Part model, mm, in its own coordinate system. A direction names the side the tool comes from. Give positions to 0.01 mm unless a question says otherwise; leave off trailing zeros. Order: outer loops, then holes, each group sorted by start corner. A loop starts at its lowest first (then second) coordinate and runs counter-clockwise, first axis right, second up. Notation, with made-up numbers: (77.25, -10) -> (135.25, -10) arc R26 cw to (135.25, 25) -> close; hole circle Ø10 at (4, 54.25). An arc over 180 degrees is marked (long way). Write item = value, one per line. Start each with the question number.
Item 1: Band-saw the part on C-C on z = 0. Write the cut outline in (x, y).
Item 2: Band-saw the part on A-A on y = 0. Write the cut outline in (x, z), plus the area to 3 significant figures.
Item 3: Pull direction Z, two halves, no side cores. Call faces 1 (the face through (29, 0, 0)), 2 (the face through (14, -5, 0)), 3 (the face through (14.703, 3.797, 15.859)): +Z half, -Z half, draft (parallel to the pull), parting line (faces both ways), or undercut.
Item 4: Band-saw the part on D-D on z = 8.5. Write the cut outline in (x, y).
Item 5: Tool access for faces 4 (the face through (31.96, -1.15, 5.73)), 5 (the face through (-1.5, -0.1, 2.5)), 6 (the face through (14.703, 3.797, -15.859)): list every direction of +Z, -Z, +X, -X, +Y, -Y with a clear straight run to the whole face (end or side of a thin tool).
Item 6: Flat gauge pins, fed straight in: P1, Ø1, axis at y = 1, z = -5, coming from the -X side; P2, Ø3, axis at x = 15, y = 3.5, coming from the -Z side. Where does each tip first touch, or does it go through?
Item 7: Drill centre lines: line 1 along X through (y, z) = (2.5, 14); line 2 along X through (y, z) = (2.5, 8); line 3 along Z through (x, y) = (12, 3.75). Where is each one in solid material? Low to high.
Item 8: Band-saw the part on B-B on x = 21. Write the cut outline in (y, z).
```python
from build123d import *

# Parameters (mm, degrees)
ESBO_O1_W                = 34
ESBO_O1_H                = 10
RESSALTO_EXTRUS_O1_DEPTH = 29
FILETE1_R                = 4
ESBO_O2_R                = 3
RESSALTO_EXTRUS_O2_DEPTH = 6
ESBO_O3_R                = 2.5
RESSALTO_EXTRUS_O3_DEPTH = 3


with BuildPart() as part:
    # Esboço1 → Ressalto-extrusão1 (new body)
    with BuildSketch(Plane(origin=(0, 0, 0), x_dir=(0, 0, -1), z_dir=(1, 0, 0))):
        Rectangle(ESBO_O1_W, ESBO_O1_H)
    extrude(amount=RESSALTO_EXTRUS_O1_DEPTH)

    # Filete1
    filete1_edges = [part.edges().sort_by_distance(p)[0] for p in [
        (14.5, 5, 17),
        (14.5, 5, -17),
    ]]
    fillet(filete1_edges, radius=FILETE1_R)

    # Esboço2 → Ressalto-extrusão2 (add)
    with BuildSketch(Plane(origin=(29, 0, 0), x_dir=(0, 0, -1), z_dir=(1, 0, 0))):
        with Locations((-8.5, 0)):
            Circle(ESBO_O2_R)
        with Locations((8.5, 0)):
            Circle(ESBO_O2_R)
    extrude(amount=RESSALTO_EXTRUS_O2_DEPTH)

    # Esboço3 → Ressalto-extrusão3 (add)
    with BuildSketch(Plane.ZY):
        with Locations(Location((0, 0, 0), (0, 0, 180))):
            Circle(ESBO_O3_R)
    extrude(amount=RESSALTO_EXTRUS_O3_DEPTH)


solid = part.part
```
Values found:
q1.outline = (-3, -2.5) -> (0, -2.5) -> (0, -5) -> (29, -5) -> (29, 5) -> (0, 5) -> (0, 2.5) -> (-3, 2.5) -> close
q2.outline = (-3, -2.5) -> (0, -2.5) -> (0, -17) -> (29, -17) -> (29, -11.5) -> (35, -11.5) -> (35, -5.5) -> (29, -5.5) -> (29, 5.5) -> (35, 5.5) -> (35, 11.5) -> (29, 11.5) -> (29, 17) -> (0, 17) -> (0, 2.5) -> (-3, 2.5) -> close
q2.area = 1,070 mm^2
q3.face_1 = undercut
q3.face_2 = draft
q3.face_3 = +Z half
q4.outline = (0, -5) -> (29, -5) -> (29, -3) -> (35, -3) -> (35, 3) -> (29, 3) -> (29, 5) -> (0, 5) -> close
q5.face_4 = +X
q5.face_5 = -X
q5.face_6 = -Z, +X, -X, +Y
q6.P1 = 0
q6.P2 = -16.87
q7.line_1 = 0 to 29
q7.line_2 = 0 to 35
q7.line_3 = -15.9 to 15.9
q8.outline = (-5, -17) -> (1, -17) arc R4 ccw to (5, -13) -> (5, 13) arc R4 ccw to (1, 17) -> (-5, 17) -> close
